The model under review builds one solid part; all positions refer to its coordinate system, in mm. Face numbers are marked on the shaded views. A direction names the side the tool comes from. Coordinates: 2 decimals unless noted, no trailing zeros. Loops run counter-clockwise (first coordinate to the right, second up) from the corner with the lowest first, then second, coordinate; pieces in that order, holes last. Notation, with made-up numbers: M -5,18.5 L 50,18.5 A10 cw 50,25.5 Z; hole C 58,89.25 d8. An arc over 180 degrees is marked long. Use one line per item in the form item = value.
```python
from build123d import *

# Parameters (mm, degrees)
MAIN_SKETCH_W                                    = 52
MAIN_SKETCH_H                                    = 40.5
MAIN_EXTRUSION_DEPTH                             = 120
MAIN_HOLE_START                                  = -112
MAIN_HOLE_SKETCH_W                               = 46
MAIN_HOLE_SKETCH_H                               = 34.5
MAIN_HOLE_DEPTH                                  = 112
FRAISAGE_POUR_VIS_T_TE_FRAIS_E_M2_51_D           = 2.9
FRAISAGE_POUR_VIS_T_TE_FRAIS_E_M2_51_CSINK_D     = 5.5
FRAISAGE_POUR_VIS_T_TE_FRAIS_E_M2_51_CSINK_ANGLE = 90
ESQUISSE6_W                                      = 10
ESQUISSE6_H                                      = 20.5
ENL_V_MAT_EXTRU_3_DEPTH                          = 133.340706134
ESQUISSE7_W                                      = 32
ESQUISSE7_H                                      = 85
ENL_V_MAT_EXTRU_4_DEPTH                          = 130.291337684
R_P_TITION_LIN_AIRE1_COUNT                       = 5
R_P_TITION_LIN_AIRE1_PITCH                       = 20
ENL_V_MAT_EXTRU_5_DEPTH                          = 130.291337684
ESQUISSE10_R                                     = 7.5
ENL_V_MAT_EXTRU_7_DEPTH                          = 4
FRAISAGE_POUR_VIS_T_TE_FRAIS_E_M2_52_D           = 2.9
FRAISAGE_POUR_VIS_T_TE_FRAIS_E_M2_52_CSINK_D     = 5.5
FRAISAGE_POUR_VIS_T_TE_FRAIS_E_M2_52_CSINK_ANGLE = 90
R_P_TITION_LIN_AIRE3_COUNT                       = 2
R_P_TITION_LIN_AIRE3_PITCH                       = 28
ENL_V_MAT_EXTRU_8_REACH                          = 126.443
ESQUISSE13_R                                     = 2.5


with BuildPart() as part:
    # Main-Sketch → Main-Extrusion (new body)
    with BuildSketch(Plane.XY):
        Rectangle(MAIN_SKETCH_W, MAIN_SKETCH_H)
    extrude(amount=MAIN_EXTRUSION_DEPTH)

    # Main-Hole-Sketch → Main-Hole (cut)
    with BuildSketch(Plane(origin=(0, 0, 0), x_dir=(-1, 0, 0), z_dir=(0, 0, -1)).offset(MAIN_HOLE_START)):
        Rectangle(MAIN_HOLE_SKETCH_W, MAIN_HOLE_SKETCH_H)
    extrude(amount=MAIN_HOLE_DEPTH, mode=Mode.SUBTRACT)

    # Fraisage pour vis à tête fraisée M2.51 (through all)
    with Locations(Plane(origin=(26, 0, 0), x_dir=(0, 0, -1), z_dir=(1, 0, 0))):
        with Locations((-10, 0)):
            CounterSinkHole(FRAISAGE_POUR_VIS_T_TE_FRAIS_E_M2_51_D / 2, FRAISAGE_POUR_VIS_T_TE_FRAIS_E_M2_51_CSINK_D / 2, counter_sink_angle=FRAISAGE_POUR_VIS_T_TE_FRAIS_E_M2_51_CSINK_ANGLE)

    # Esquisse6 → Enlèv. mat.-Extru.3 (cut, through all)
    with BuildSketch(Plane(origin=(26, 0, 0), x_dir=(0, 0, -1), z_dir=(1, 0, 0))):
        with Locations((-100, 0)):
            Rectangle(ESQUISSE6_W, ESQUISSE6_H)
    enl_v_mat_extru_3 = extrude(amount=-ENL_V_MAT_EXTRU_3_DEPTH, mode=Mode.SUBTRACT)

    # Esquisse7 → Enlèv. mat.-Extru.4 (cut, through all)
    with BuildSketch(Plane(origin=(0, 20.25, 0), x_dir=(1, 0, 0), z_dir=(0, 1, 0))):
        with Locations((0, -62.5)):
            Rectangle(ESQUISSE7_W, ESQUISSE7_H)
    extrude(amount=-ENL_V_MAT_EXTRU_4_DEPTH, mode=Mode.SUBTRACT)

    # Répétition linéaire1: Enlèv. mat.-Extru.3 ×5
    with Locations(*[(0, 0, -i * R_P_TITION_LIN_AIRE1_PITCH) for i in range(1, R_P_TITION_LIN_AIRE1_COUNT)]):
        add(enl_v_mat_extru_3, mode=Mode.SUBTRACT)

    # Esquisse8 → Enlèv. mat.-Extru.5 (cut, through all)
    with BuildSketch(Plane(origin=(0, 20.25, 0), x_dir=(-1, 0, 0), z_dir=(0, 1, 0))):
        Polygon((-19.5, 120), (-26, 113.5), (-26, 120), align=None)
    extrude(amount=-ENL_V_MAT_EXTRU_5_DEPTH, mode=Mode.SUBTRACT)

    # Esquisse10 → Enlèv. mat.-Extru.7 (cut)
    with BuildSketch(Plane.XY.offset(120)):
        with Locations((-31, 0)):
            Circle(ESQUISSE10_R)
    extrude(amount=-ENL_V_MAT_EXTRU_7_DEPTH, mode=Mode.SUBTRACT)

    # Fraisage pour vis à tête fraisée M2.52 (through all)
    with Locations(Plane(origin=(26, 0, 0), x_dir=(0, 0, -1), z_dir=(1, 0, 0))):
        with Locations((-3, 15.25)):
            fraisage_pour_vis_t_te_frais_e_m2_52 = CounterSinkHole(FRAISAGE_POUR_VIS_T_TE_FRAIS_E_M2_52_D / 2, FRAISAGE_POUR_VIS_T_TE_FRAIS_E_M2_52_CSINK_D / 2, counter_sink_angle=FRAISAGE_POUR_VIS_T_TE_FRAIS_E_M2_52_CSINK_ANGLE)

    # Répétition linéaire3: Fraisage pour vis à tête fraisée M2.52 ×2
    with Locations(*[(0, -i * R_P_TITION_LIN_AIRE3_PITCH, 0) for i in range(1, R_P_TITION_LIN_AIRE3_COUNT)]):
        add(fraisage_pour_vis_t_te_frais_e_m2_52, mode=Mode.SUBTRACT)

    # Esquisse13 → Enlèv. mat.-Extru.8 (cut, up to next)
    with BuildSketch(Plane.XY.offset(120), mode=Mode.PRIVATE) as enl_v_mat_extru_8_sk1:
        with Locations((-3.25, 0)):
            Circle(ESQUISSE13_R)
    enl_v_mat_extru_8_tool1 = extrude(enl_v_mat_extru_8_sk1.sketch, amount=-ENL_V_MAT_EXTRU_8_REACH, mode=Mode.PRIVATE) & part.part
    add(enl_v_mat_extru_8_tool1.solids().sort_by_distance((-3.25, 0, 120))[0], mode=Mode.SUBTRACT)


solid = part.part
```
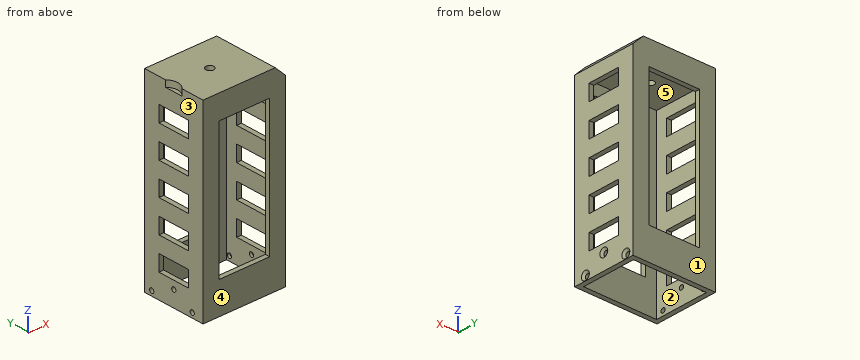
1. Wall thickness on line 1 along Y through (x, z) = (23.75, 3); line 2 along Y through (x, z) = (20, 60); line 3 along Y through (x, z) = (24.5, 38.5): over which ranges is each line inside the solid? List them lowest first. Write a range as from..to.
Response values:
line_1 = -20.25..-14.2, -11.3..13.8, 16.7..20.25
line_2 = -20.25..-17.25, 17.25..20.25
line_3 = -20.25..-10.25, 10.25..20.25
2. Add section A-A (z = 18.5). State the section outline as (x, y) points.
Response values:
outline = M -26,-20.25 L 26,-20.25 L 26,-10.25 L 23,-10.25 L 23,-17.25 L -23,-17.25 L -23,-10.25 L -26,-10.25 Z; M -26,10.25 L -23,10.25 L -23,17.25 L 23,17.25 L 23,10.25 L 26,10.25 L 26,20.25 L -26,20.25 Z
3. The part is to be moulded in two halves that separate along X. For the marked faces 1, 2 and 3, say which applies: pulls with the +X half, pulls with the -X half, needs draft (parallel to the pull), parting line crosses it, or undercut.
Response values:
face_1 = needs draft
face_2 = undercut
face_3 = pulls with the -X half
4. Add section C-C (y = 15.25). State the section outline as (x, z) points.
Response values:
outline = M -26,0 L -23,0 L -23,1.55 L -26,1.55 Z; M -26,4.45 L -23,4.45 L -23,112 L 23,112 L 23,4.45 L 24.7,4.45 L 26,5.75 L 26,113.5 L 19.5,120 L -26,120 Z; M 23,0 L 26,0 L 26,0.25 L 24.7,1.55 L 23,1.55 Z
5. Machinability: for the marked faces 4 and 5, which of the approach directions +Z, -Z, +X, -X, +Y, -Y give a long, thin tool a straight path to every point of the face, cutting with its end or side? Answer none if there is none.
Response values:
face_4 = +Z, -Z, +X, -X, -Y
face_5 = -Z
6. Insertion check: P1, Ø3.5, axis at y = 0, z = 10, coming from the +X side; P2, Ø3.5, axis at x = -24.5, y = 3.5, coming from the +Z side; P3, Ø1.5, axis at x = 24.5, y = 4.5, coming from the +Z side; P4, Ø1, axis at x = -17, y = -15, coming from the -Z side. Each pin has a flat end and moves straight along its axis. Give the tip position at first contact, or say it passes through.
Response values:
P1 = 25
P2 = 120
P3 = 115.75
P4 = 112
7. Add section D-D (z = 42). State the section outline as (x, y) points.
Response values:
outline = M -26,-20.25 L -16,-20.25 L -16,-17.25 L -23,-17.25 L -23,-10.25 L -26,-10.25 Z; M -26,10.25 L -23,10.25 L -23,17.25 L -16,17.25 L -16,20.25 L -26,20.25 Z; M 16,-20.25 L 26,-20.25 L 26,-10.25 L 23,-10.25 L 23,-17.25 L 16,-17.25 Z; M 16,17.25 L 23,17.25 L 23,10.25 L 26,10.25 L 26,20.25 L 16,20.25 Z
8. Add section B-B (x = -3.25). State the section outline as (y, z) points.
Response values:
outline = M -20.25,0 L -17.25,0 L -17.25,20 L -20.25,20 Z; M -20.25,105 L -17.25,105 L -17.25,112 L -2.5,112 L -2.5,120 L -20.25,120 Z; M 2.5,112 L 17.25,112 L 17.25,105 L 20.25,105 L 20.25,120 L 2.5,120 Z; M 17.25,0 L 20.25,0 L 20.25,20 L 17.25,20 Z
